from build123d import *

# Parameters (mm, degrees)
SKETCH1_R                = 15
BOSS_EXTRUDE1_DEPTH      = 3
CHAMFER1_SIZE            = 2
M5_CLEARANCE_HOLE1_D     = 5.8
M5_CLEARANCE_HOLE1_DEPTH = 6
M5_CLEARANCE_HOLE1_TIP   = 1.742495795


with BuildPart() as part:
    # Sketch1 → Boss-Extrude1 (new body)
    with BuildSketch(Plane(origin=(0, 0, 0), x_dir=(1, 0, 0), z_dir=(0, 1, 0))):
        Circle(SKETCH1_R)
    extrude(amount=BOSS_EXTRUDE1_DEPTH)

    # Chamfer1
    chamfer1_edges = [part.edges().sort_by_distance(p)[0] for p in [
        (-15, 3, 0),
    ]]
    chamfer(chamfer1_edges, length=CHAMFER1_SIZE)

    # M5 Clearance Hole1
    with Locations(Plane(origin=(0, 3, 0), x_dir=(1, 0, 0), z_dir=(0, 1, 0))):
        with Locations((0, 0)):
            Hole(M5_CLEARANCE_HOLE1_D / 2, depth=M5_CLEARANCE_HOLE1_DEPTH)
            with Locations((0, 0, -(M5_CLEARANCE_HOLE1_DEPTH + M5_CLEARANCE_HOLE1_TIP / 2))):  # 118° drill point
                Cone(0, M5_CLEARANCE_HOLE1_D / 2, M5_CLEARANCE_HOLE1_TIP, mode=Mode.SUBTRACT)


solid = part.part
Work out the finished part from the listing and answer in its coordinate system (mm). Give positions to 0.01 mm unless a question says otherwise; leave off trailing zeros. Write each loop counter-clockwise with the first axis right and the second up, starting at its lowest first coordinate (ties: lowest second). Pieces come first, ordered by that corner, then holes.
Q1. Straight lines are drawn through the part: L1, parallel to Z at x = 0, y = 0.8; L2, parallel to Z at x = 0, y = 2.4; L3, parallel to X at y = 1.7, z = 2.25. For each, find the intervals that lie inside material, in ascending order.
Answer:
L1: z = -15 to -2.9, 2.9 to 15
L2: z = -13.6 to -2.9, 2.9 to 13.6
L3: x = -14.12 to -1.83, 1.83 to 14.12
Q2. The part is cut by section C-C on y = 0.6. Give the vertices of the cut face in (x, z).
Answer:
outline: circle Ø30 at (0, 0); hole circle Ø5.8 at (0, 0)
Q3. The part is cut by section B-B on x = 0. Give the vertices of the cut face in (y, z), and give its area (3 significant figures).
Answer:
outline: (0, -15) - (1, -15) - (3, -13) - (3, -2.9) - (0, -2.9) - close; (0, 2.9) - (3, 2.9) - (3, 13) - (1, 15) - (0, 15) - close
area: 68.6 mm2
Q4. For a pull along Z with two mould halves and no side action, classify faces 1 (the face through (-14.985, 0.493, -0.66)), 2 (the face through (2.9, 1.5, -0.1)), 3 (the face through (-0.2, 3, -3.1)) as released by +Z, released by -Z, zero draft, split by the parting line, or undercut.
Answer:
face 1: split by the parting line
face 2: undercut
face 3: zero draft
Q5. The part is cut by section D-D on y = 2.3. Give the vertices of the cut face in (x, z), and give its area (3 significant figures).
Answer:
outline: circle Ø27.4 at (0, 0); hole circle Ø5.8 at (0, 0)
area: 563 mm2
Q6. The part is cut by section A-A on z = 0. Give the vertices of the cut face in (x, y), and give its area (3 significant figures).
Answer:
outline: (-15, 0) - (-2.9, 0) - (-2.9, 3) - (-13, 3) - (-15, 1) - close; (2.9, 0) - (15, 0) - (15, 1) - (13, 3) - (2.9, 3) - close
area: 68.6 mm2
